Source: CAD feature listing. Evaluate the final solid. Frame: model axes, mm. Give positions to 0.01 mm unless a question says otherwise; leave off trailing zeros. Loops run counter-clockwise (first coordinate to the right, second up) from the corner with the lowest first, then second, coordinate; pieces in that order, holes last. Notation, with made-up numbers: (37.5, 23) - (46.5, 23) arc R22 ccw to (46.5, 61) - close; hole circle Ø10 at (7.25, 71.25). An arc over 180 degrees is marked (long way). Put each result on its own line as item: value.
```python
from build123d import *

# Parameters (mm, degrees)
SKETCH1_R           = 1.6
BOSS_EXTRUDE1_DEPTH = 3


with BuildPart() as part:
    # Sketch1 → Boss-Extrude1 (new body)
    with BuildSketch(Plane.XY):
        with BuildLine():
            Line((-36.934217786, 0), (-30.434217786, 0))
            ThreePointArc((-30.434217786, 0), (-19.491470952, 40.838887158), (10.404669372, 70.735027482))
            ThreePointArc((10.404669372, 70.735027482), (20.808844345, 88.613000102), (10.652125885, 106.632706869))
            Line((10.652125885, 106.632706869), (7.324830428, 101.048881572))
            ThreePointArc((7.324830428, 101.048881572), (14.308998775, 88.657806037), (7.154669372, 76.364192606))
            ThreePointArc((7.154669372, 76.364192606), (-25.120636077, 44.088887158), (-36.934217786, 0))
        make_face()
        with Locations((12.048125899, 103.114840794)):
            Circle(SKETCH1_R, mode=Mode.SUBTRACT)
        with Locations((-10.337645521, 56.751553408)):
            Circle(SKETCH1_R, mode=Mode.SUBTRACT)
        with Locations((-31.900795415, 10)):
            Circle(SKETCH1_R, mode=Mode.SUBTRACT)
    extrude(amount=BOSS_EXTRUDE1_DEPTH)


solid = part.part
```
1) Mould query, pull axis Y, two halves, no side actions, for faces 1 (the cylindrical face through (20.805, 88.31, 1.479)), 2 (the cylindrical face through (-11.936, 56.822, 1.479)), 3 (the flat face through (-12, 54, 3)), 4 (the cylindrical face through (12.786, 101.695, 1.479)). Classes: pulls with the +Y half, pulls with the -Y half, needs draft (parallel to the pull), parting line crosses it, or undercut.
Check result:
face 1: parting line crosses it
face 2: undercut
face 3: needs draft
face 4: undercut
2) Pin query (flat end, axial travel): P1, Ø1, axis at x = -3.5, z = 2, coming from the +Y side; P2, Ø1, axis at y = 60, z = 2, coming from the +X side. Return the tip coordinate at first contact, or that it passes through.
Check result:
P1: y = 69.52
P2: x = -3.63
3) Section query A-A, the plane y = 10. Output: boundary loops of the cut face in (x, z).
Check result:
outline: (-36.37, 0) - (-33.5, 0) - (-33.5, 3) - (-36.37, 3) - close; (-30.3, 0) - (-29.82, 0) - (-29.82, 3) - (-30.3, 3) - close
4) Section query B-B, the plane z = 2.4. Output: boundary loops of the cut face in (x, y).
Check result:
outline: (-36.93, 0) - (-30.43, 0) arc R81.68 cw to (10.4, 70.74) arc R20.81 ccw to (10.65, 106.63) - (7.32, 101.05) arc R14.31 cw to (7.15, 76.36) arc R88.18 ccw to start; hole circle Ø3.2 at (-31.9, 10); hole circle Ø3.2 at (-10.34, 56.75); hole circle Ø3.2 at (12.05, 103.11)
5) Material intervals for line 1 along Y through (x, z) = (10, 1.05); line 2 along X through (y, z) = (38, 2.3); line 3 along X through (y, z) = (11, 2), sorted ascending. Write a range as [from, to].
Check result:
line 1: [70.5, 78.52], [98.99, 105.54]
line 2: [-28.33, -21.06]
line 3: [-36.25, -33.15], [-30.65, -29.69]
6) Section query C-C, the plane x = -28. Output: boundary loops of the cut face in (y, z).
Check result:
outline: (19.79, 0) - (38.68, 0) - (38.68, 3) - (19.79, 3) - close
7) Section query D-D, the plane y = 39. Output: boundary loops of the cut face in (x, z).
Check result:
outline: (-27.84, 0) - (-20.52, 0) - (-20.52, 3) - (-27.84, 3) - close
